Verification items for the finished model (mm, model axes). Face numbers are marked on the shaded views. Give positions to 0.01 mm unless a question says otherwise; leave off trailing zeros. Order: outer loops, then holes, each group sorted by start corner. A loop starts at its lowest first (then second) coordinate and runs counter-clockwise, first axis right, second up. Notation, with made-up numbers: (88.5, 24.25) -> (145.5, 24.25) arc R4 cw to (145.5, 29.25) -> close; hole circle Ø1 at (-5.75, 1.25). An arc over 180 degrees is marked (long way). One line per question, with ' | ' between items. Start each with the question number.
Q1. Section check B-B on x = -5. Record the cut outline in (y, z).
Q2. Mould release check, pull along X, two halves, no side actions. Record for the marked faces 1, 2, 3 and 4: released by +X, released by -X, zero draft, split by the parting line, or undercut.
Q3. Section check A-A on z = 0. Record the cut outline in (x, y).
Q4. Material ranges on probe 1 along X at (y, z) = (6.5, 10); probe 2 along Z at (x, y) = (5, 4.25); probe 3 along Z at (x, y) = (4, 4), recorded low to high. Write a range as [from, to].
Q5. Go/stop test with a flat-tipped pin: pin 1 (4 mm diameter, centred on x = 5, z = 10, fed in from -Y). Record where the tip stops, or that it passes through.
Q6. Section check C-C on y = 5. Record the cut outline in (x, z).
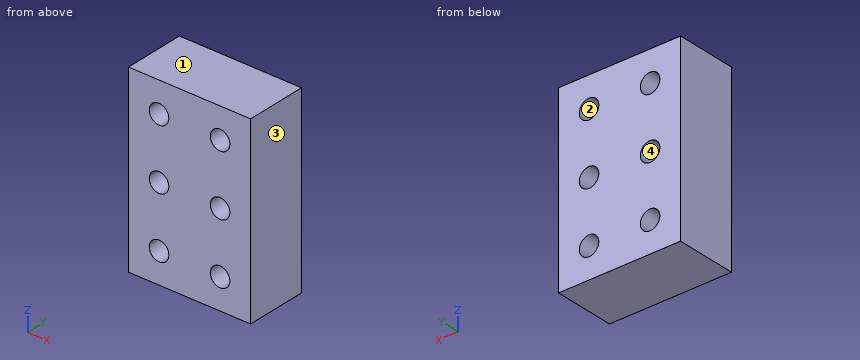
from build123d import *

# Parameters (mm, degrees)
SKETCH_1_W      = 20
SKETCH_1_H      = 30
SKETCH_1_R      = 1.6
EXTRUDE_1_DEPTH = 10


with BuildPart() as part:
    # 草图1 → 凸台-拉伸1 (new body)
    with BuildSketch(Plane(origin=(0, 0, 0), x_dir=(1, 0, 0), z_dir=(0, 1, 0))):
        Rectangle(SKETCH_1_W, SKETCH_1_H)
        with Locations(Location((-5, 0, 0), (0, 0, 270))):
            Circle(SKETCH_1_R, mode=Mode.SUBTRACT)
        with Locations(Location((-5, 10, 0), (0, 0, 270))):
            Circle(SKETCH_1_R, mode=Mode.SUBTRACT)
        with Locations(Location((-5, -10, 0), (0, 0, 270))):
            Circle(SKETCH_1_R, mode=Mode.SUBTRACT)
        with Locations(Location((5, -10, 0), (0, 0, 90))):
            Circle(SKETCH_1_R, mode=Mode.SUBTRACT)
        with Locations(Location((5, 0, 0), (0, 0, 90))):
            Circle(SKETCH_1_R, mode=Mode.SUBTRACT)
        with Locations(Location((5, 10, 0), (0, 0, 90))):
            Circle(SKETCH_1_R, mode=Mode.SUBTRACT)
    extrude(amount=EXTRUDE_1_DEPTH)


solid = part.part
Filled in:
1) outline: (0, -15) -> (10, -15) -> (10, -11.6) -> (0, -11.6) -> close; (0, -8.4) -> (10, -8.4) -> (10, -1.6) -> (0, -1.6) -> close; (0, 1.6) -> (10, 1.6) -> (10, 8.4) -> (0, 8.4) -> close; (0, 11.6) -> (10, 11.6) -> (10, 15) -> (0, 15) -> close
2) face 1: zero draft | face 2: undercut | face 3: released by +X | face 4: undercut
3) outline: (-10, 0) -> (-6.6, 0) -> (-6.6, 10) -> (-10, 10) -> close; (-3.4, 0) -> (3.4, 0) -> (3.4, 10) -> (-3.4, 10) -> close; (6.6, 0) -> (10, 0) -> (10, 10) -> (6.6, 10) -> close
4) probe 1: [-10, -6.6], [-3.4, 3.4], [6.6, 10] | probe 2: [-15, -11.6], [-8.4, -1.6], [1.6, 8.4], [11.6, 15] | probe 3: [-15, -11.25], [-8.75, -1.25], [1.25, 8.75], [11.25, 15]
5) pin 1: y = 0
6) outline: (-10, -15) -> (10, -15) -> (10, 15) -> (-10, 15) -> close; hole circle Ø3.2 at (-5, -10); hole circle Ø3.2 at (-5, 0); hole circle Ø3.2 at (-5, 10); hole circle Ø3.2 at (5, -10); hole circle Ø3.2 at (5, 0); hole circle Ø3.2 at (5, 10)
